Can you work these out from the model? Positions are in its coordinate system, mm. A direction names the side the tool comes from. Round coordinates to 2 decimals unless told otherwise and drop trailing zeros. Write each loop counter-clockwise with the first axis right and the second up, starting at its lowest first coordinate (ties: lowest second). Pieces come first, ordered by that corner, then holes. Notation, with made-up numbers: M 29,-37.5 L 58,-37.5 A28 cw 58,-3.5 Z; hole C 22.25,76 d6. An arc over 180 degrees is marked long. Answer in a Markdown table with one row per item. Add a question column.
(1) For faces 1 (the face through (37, -2, 10)), 2 (the face through (23.866, -38.778, 10.004)), 3 (the face through (37, -41.5, 13)), 4 (the face through (5, -22, 15.5)), which set-ups out of +Z, -Z, +X, -X, +Y, -Y let a thin tool reach every point of the face, with its end or its side?
(2) Suppose I cut it at A-A, the plane z = 8.5. Write out the boundary of the cut face in (x, y), then the cut area to 3 significant figures.
(3) Suppose I cut it at B-B, the plane x = 66. Write out the boundary of the cut face in (y, z).
(4) I'm going to push flat-ended pins straight in: pin 1 (1 mm diameter, centred on x = 25, y = -43.5, fed in from +Z); pin 2 (12 mm diameter, centred on x = 59.5, y = -29, fed in from -Z); pin 3 (5 mm diameter, centred on x = 49, z = 14, fed in from -Y); pin 4 (8 mm diameter, centred on x = 4.5, y = -20, fed in from +Z). Where does each tip first touch, or does it pass through?
(5) If I drill on probe 1 along X at (y, z) = (-7.5, 6.75); probe 2 along Y at (x, z) = (22.2, 12.5); probe 3 along X at (y, z) = (-6, 5.5), over which ranges is the centre line in solid material (lowest first)?
(6) Suppose I cut it at C-C, the plane y = -16. Write out the boundary of the cut face in (x, z), then the cut area to 3 significant figures.
(7) If we mould it in two halves opening along X, with no side actions, what happens to faces 5 (the face through (53.748, -6.081, 10.004)), 6 (the face through (37, -43, 10)), 7 (the face through (0, -23, 8))? For each: released by +X, released by -X, zero draft, split by the parting line, or undercut.
from build123d import *

# Parameters (mm, degrees)
SKETCH_1_W                   = 74.4
SKETCH_1_H                   = 45
EXTRUDE_1_DEPTH              = 10
SKETCH_2_W                   = 74.4
SKETCH_2_H                   = 38
EXTRUDE_2_DEPTH              = 6.5
HOLE_WIZARD_M5_1_D           = 4.2
HOLE_WIZARD_M5_1_DEPTH       = 12.4
HOLE_WIZARD_M5_1_CSINK_D     = 5.05
HOLE_WIZARD_M5_1_CSINK_ANGLE = 90
HOLE_WIZARD_M5_1_TIP         = 1.2618073
SKETCH_5_OUTSIDE_W           = 94.1
SKETCH_5_OUTSIDE_H           = 64.7
SKETCH_5_OUTSIDE_W_2         = 54
SKETCH_5_OUTSIDE_H_2         = 38
CUT_EXTRUDE_1_DEPTH          = 1


with BuildPart() as part:
    # 草图1 → 凸台-拉伸1 (new body)
    with BuildSketch(Plane.XY):
        with Locations((37.2, -22.5)):
            Rectangle(SKETCH_1_W, SKETCH_1_H)
    extrude(amount=EXTRUDE_1_DEPTH)

    # 草图2 → 凸台-拉伸2 (add)
    with BuildSketch(Plane.XY.offset(10)):
        with Locations((37.2, -22.5)):
            Rectangle(SKETCH_2_W, SKETCH_2_H)
    extrude(amount=EXTRUDE_2_DEPTH)

    # M5 螺纹孔1
    with Locations(Plane.XY.offset(16.5)):
        with Locations((22.2, -7.5), (52.2, -7.5), (52.2, -37.5), (22.2, -37.5)):
            CounterSinkHole(HOLE_WIZARD_M5_1_D / 2, HOLE_WIZARD_M5_1_CSINK_D / 2, depth=HOLE_WIZARD_M5_1_DEPTH, counter_sink_angle=HOLE_WIZARD_M5_1_CSINK_ANGLE)
            with Locations((0, 0, -(HOLE_WIZARD_M5_1_DEPTH + HOLE_WIZARD_M5_1_TIP / 2))):  # 118° drill point
                Cone(0, HOLE_WIZARD_M5_1_D / 2, HOLE_WIZARD_M5_1_TIP, mode=Mode.SUBTRACT)

    # 草图5 outside → 切除-拉伸1 (cut)
    with BuildSketch(Plane.XY.offset(16.5)):
        with Locations((37.2, -22.5)):
            Rectangle(SKETCH_5_OUTSIDE_W, SKETCH_5_OUTSIDE_H)
        with Locations((37.2, -22.5)):
            Rectangle(SKETCH_5_OUTSIDE_W_2, SKETCH_5_OUTSIDE_H_2, mode=Mode.SUBTRACT)
    extrude(amount=-CUT_EXTRUDE_1_DEPTH, mode=Mode.SUBTRACT)


solid = part.part
Calculated:
| question | item | result |
|---|---|---|
| 1 | face 1 | +Z, +X, -X, +Y |
| 1 | face 2 | +Z |
| 1 | face 3 | +Z, +X, -X, -Y |
| 1 | face 4 | +Z, -X, +Y, -Y |
| 2 | outline | M 0,-45 L 74.4,-45 L 74.4,0 L 0,0 Z; hole C 22.2,-37.5 d4.2; hole C 22.2,-7.5 d4.2; hole C 52.2,-37.5 d4.2; hole C 52.2,-7.5 d4.2 |
| 2 | area | 3,290 mm² |
| 3 | outline | M -45,0 L 0,0 L 0,10 L -3.5,10 L -3.5,15.5 L -41.5,15.5 L -41.5,10 L -45,10 Z |
| 4 | pin 1 | z = 10 |
| 4 | pin 2 | z = 0 |
| 4 | pin 3 | y = -41.5 |
| 4 | pin 4 | z = 15.5 |
| 5 | probe 1 | 0 to 20.1, 24.3 to 50.1, 54.3 to 74.4 |
| 5 | probe 2 | -41.5 to -39.6, -35.4 to -9.6, -5.4 to -3.5 |
| 5 | probe 3 | 0 to 20.73, 23.67 to 50.73, 53.67 to 74.4 |
| 6 | outline | M 0,0 L 74.4,0 L 74.4,15.5 L 64.2,15.5 L 64.2,16.5 L 10.2,16.5 L 10.2,15.5 L 0,15.5 Z |
| 6 | area | 1,210 mm² |
| 7 | face 5 | undercut |
| 7 | face 6 | zero draft |
| 7 | face 7 | released by -X |
